from build123d import *

# Parameters (mm, degrees)
F1_DEPTH       = 17.78
F2_W           = 22.352
F2_H           = 7.714197
F2_H_2         = 6.145762
F3_DEPTH       = 12.701
F4_R           = 3.048
F6_D           = 4.2672
F6_CSINK_D     = 8.5852
F6_CSINK_ANGLE = 100


with BuildPart() as f1:
    # F0 (on Front) → F1 (new body)
    with BuildSketch(Plane.XZ):
        Polygon((15.748, -12.7), (15.748, 0), (-28.702, 0), (-28.702, -6.35), (0, -6.35), (0, -12.7), align=None)
    extrude(amount=F1_DEPTH)

    # F2 (on face) → F3 (cut, through all)
    with BuildSketch(Plane.XY):
        with Locations((-11.176, -18.589098)):
            Rectangle(F2_W, F2_H)
        with Locations((-11.176, 0.024881)):
            Rectangle(F2_W, F2_H_2)
    extrude(amount=-F3_DEPTH, mode=Mode.SUBTRACT)

    # F4
    f4_edges = [f1.edges().sort_by_distance(p)[0] for p in [
        (15.748, 0, -6.35),
        (15.748, -17.78, -6.35),
    ]]
    fillet(f4_edges, radius=F4_R)

    # F6 (through all)
    with Locations(Plane.XY):
        with Locations((7.112, -8.89)):
            CounterSinkHole(F6_D / 2, F6_CSINK_D / 2, counter_sink_angle=F6_CSINK_ANGLE)


solid = f1.part
Model file for the job. Use its own axes, mm. A direction names the side the tool comes from. Give positions to 0.01 mm unless a question says otherwise; leave off trailing zeros. Loops run counter-clockwise (first coordinate to the right, second up) from the corner with the lowest first, then second, coordinate; pieces in that order, holes last. Notation, with made-up numbers: (-3, 86) -> (1, 86) arc R18 ccw to (1, 110) -> close; hole circle Ø2 at (-23.5, 79). An arc over 180 degrees is marked (long way). Use a Markdown table: item, result. Add a question column.
(1) Slice it at B-B on z = -2.75. List the corners of the cut face in (x, y).
(2) Slice it at C-C on x = -17.5. List the corners of the cut face in (y, z).
(3) Tool access for faces 5 (the flat face through (-11, -14.732, -3)), 6 (the flat face through (-15, -9, -6.35)), 7 (the flat face through (-26, -17.78, -3)), 8 (the flat face through (-22.352, -2, -3)): list every direction of +Z, -Z, +X, -X, +Y, -Y with a clear straight run to the whole face (end or side of a thin tool).
(4) Mould opens along Y. For faces 1 (the cylindrical face through (7.575, -10.973, -7.332)), 2 (the flat face through (-28.702, -9, -3)), 3 (the flat face through (6, -17.78, -6)), 4 (the flat face through (-26, 0, -3)) say: +Y half, -Y half, draft (parallel to the pull), parting line (faces both ways), or undercut.
(5) Wall check: line 1 along X through (y, z) = (-8.89, -7); line 2 along Z through (x, y) = (-22, -13); line 3 along Y through (x, z) = (-4, -2.25). Give the ranges that are in metal, low to high.
(6) Drop flat-ended pins along their axis: pin 1 Ø1.5 at (y, z) = (-16.5, -4) entering from +X; pin 2 Ø9 at (x, y) = (-14, -10) entering from -Z; pin 3 Ø7 at (x, y) = (7.112, -8.89) entering from +Z; pin 4 Ø1 at (y, z) = (-3.5, -6.5) entering from -X. Give the stop position or say it passes through.
(7) Slice it at A-A on y = -8.89. List the corners of the cut face in (x, z).
Filled sheet:
| question | item | result |
|---|---|---|
| 1 | outline | (-28.7, -17.78) -> (-22.35, -17.78) -> (-22.35, -14.73) -> (0, -14.73) -> (0, -17.78) -> (12.7, -17.78) arc R3.05 ccw to (15.75, -14.73) -> (15.75, -3.05) arc R3.05 ccw to (12.7, 0) -> (0, 0) -> (0, -3.05) -> (-22.35, -3.05) -> (-22.35, 0) -> (-28.7, 0) -> close; hole circle Ø4.27 at (7.11, -8.89) |
| 2 | outline | (-14.73, -6.35) -> (-3.05, -6.35) -> (-3.05, 0) -> (-14.73, 0) -> close |
| 3 | face 5 | +Z, -Z, -Y |
| 3 | face 6 | -Z, -X, +Y, -Y |
| 3 | face 7 | +Z, -Z, +X, -X, -Y |
| 3 | face 8 | +Z, -Z, +Y |
| 4 | face 1 | undercut |
| 4 | face 2 | draft |
| 4 | face 3 | -Y half |
| 4 | face 4 | +Y half |
| 5 | line 1 | 0 to 4.98, 9.25 to 15.75 |
| 5 | line 2 | -6.35 to 0 |
| 5 | line 3 | -14.73 to -3.05 |
| 6 | pin 1 | x = 15.57 |
| 6 | pin 2 | z = -6.35 |
| 6 | pin 3 | z = -0.67 |
| 6 | pin 4 | x = -28.7 |
| 7 | outline | (-28.7, -6.35) -> (0, -6.35) -> (0, -12.7) -> (4.98, -12.7) -> (4.98, -1.81) -> (2.82, 0) -> (-28.7, 0) -> close; (9.25, -12.7) -> (15.75, -12.7) -> (15.75, 0) -> (11.4, 0) -> (9.25, -1.81) -> close |
